Can you work these out from the model? Positions are in its coordinate system, mm. Coordinates: 2 decimals unless noted, no trailing zeros. Loops run counter-clockwise (first coordinate to the right, second up) from the corner with the lowest first, then second, coordinate; pieces in that order, holes last. Notation, with made-up numbers: M -11.75,84 L 33.25,84 A21 ccw 33.25,105 Z; hole C -3,-37 d9. An arc over 180 degrees is marked long. Return JSON: item names as keys, results as strings. Group by question number.
```python
from build123d import *

# Parameters (mm, degrees)
SKETCH1_W           = 692.15
SKETCH1_H           = 127
BOSS_EXTRUDE1_DEPTH = 44.45
FILLET1_R           = 31.75
SKETCH2_R           = 4.7625
CUT_EXTRUDE1_DEPTH  = 25.4


with BuildPart() as part:
    # Sketch1 → Boss-Extrude1 (new, symmetric)
    with BuildSketch(Plane.XY):
        Rectangle(SKETCH1_W, SKETCH1_H)
    extrude(amount=BOSS_EXTRUDE1_DEPTH, both=True)

    # Fillet1
    fillet1_edges = [part.edges().sort_by_distance(p)[0] for p in [
        (0, -63.5, 44.45),
        (0, 63.5, 44.45),
    ]]
    fillet(fillet1_edges, radius=FILLET1_R)

    # Sketch2 → Cut-Extrude1 (cut)
    with BuildSketch(Plane(origin=(0, 0, -44.45), x_dir=(-1, 0, 0), z_dir=(0, 0, -1))):
        with Locations(Location((157.967933997, 0, 0), (0, 0, 180))):
            Circle(SKETCH2_R)
        with Locations(Location((183.367933997, 0, 0), (0, 0, 180))):
            Circle(SKETCH2_R)
        with Locations((12.7, 0)):
            Circle(SKETCH2_R)
        with Locations((-12.7, 0)):
            Circle(SKETCH2_R)
        with Locations((-157.967933997, 0)):
            Circle(SKETCH2_R)
        with Locations((-183.367933997, 0)):
            Circle(SKETCH2_R)
    extrude(amount=-CUT_EXTRUDE1_DEPTH, mode=Mode.SUBTRACT)


solid = part.part
```
1) Suppose I cut it at B-B, the plane y = 43. List the corners of the cut face in (x, z) for me (3 decimals), then the cut area to 3 significant figures.
2) Suppose I cut it at A-A, the plane x = -120. List the corners of the cut face in (y, z) for me.
3) For pin 1 (5 mm diameter, centred on x = 158.5, y = 0.5, fed in from -Z), with a flat end and sliding along its axis, tell me the tip position at first contact or that it passes through.
4) If I drill on line 1 (Z direction, x = -187.5, y = -1.5); line 2 (Y direction, x = 135, z = 32.5); line 3 (Z direction, x = 109, y = -55.5), over which ranges is the centre line in solid material (lowest first)? Write a range as from..to.
5) Suppose I cut it at C-C, the plane y = -45. List the corners of the cut face in (x, z) for me (3 decimals).
Returned:
{
 "1": {"outline": "M -346.075,-44.45 L 346.075,-44.45 L 346.075,42.39 L -346.075,42.39 Z", "area": "60,100 mm²"},
 "2": {"outline": "M -63.5,-44.45 L 63.5,-44.45 L 63.5,12.7 A31.75 ccw 31.75,44.45 L -31.75,44.45 A31.75 ccw -63.5,12.7 Z"},
 "3": {"pin 1": "stops at z = -19.05"},
 "4": {"line 1": "z = -19.05..44.45", "line 2": "y = -56.57..56.57", "line 3": "z = -44.45..33.77"},
 "5": {"outline": "M -346.075,-44.45 L 346.075,-44.45 L 346.075,41.553 L -346.075,41.553 Z"}
}
